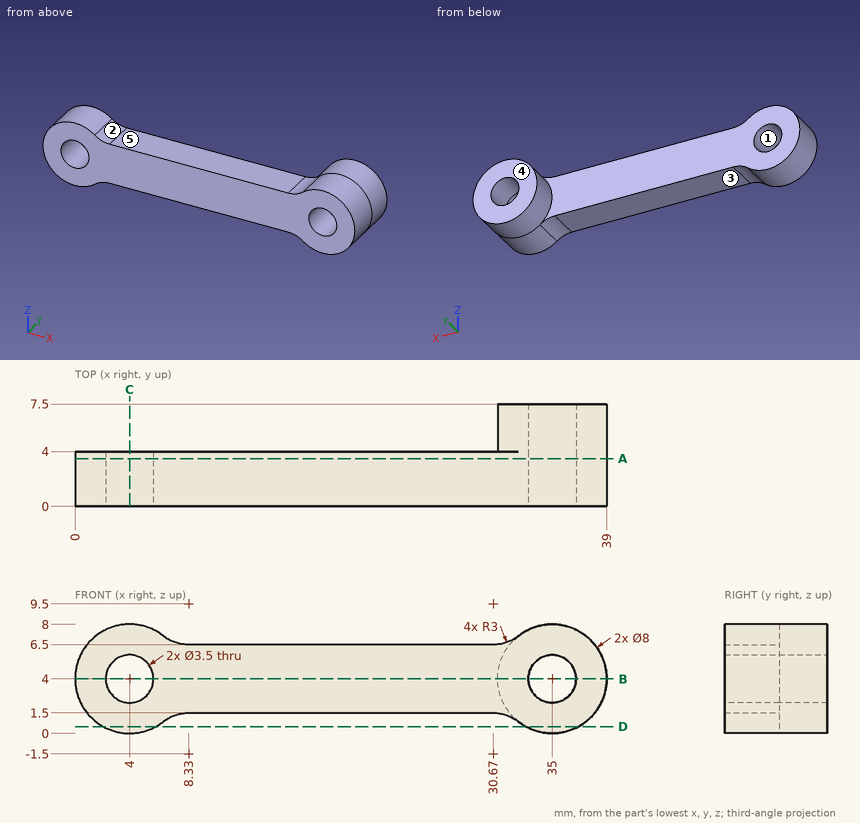
The figure shows three views and two pictorial views of one solid part (mm, origin at its lowest corner). Answer the questions. A direction names the side the tool comes from. Round coordinates to 2 decimals unless told otherwise and drop trailing zeros. Write each loop counter-clockwise with the first axis right and the second up, starting at its lowest first coordinate (ties: lowest second). Pieces come first, ordered by that corner, then holes. Notation, with made-up numbers: (15.5, 59.5) - (71.5, 59.5) arc R23 cw to (71.5, 72.5) - close; hole circle Ø7 at (1.25, 26.25). An arc over 180 degrees is marked (long way). One line per question, with ' | ' between items. Start each with the question number.
1. Section D-D (z = 0.5) is taken. Determine the outline of the cut face in (x, y), and give its area (3 significant figures).
2. Section A-A (y = 3.5) is taken. Determine the outline of the cut face in (x, z).
3. For a pull along X with two mould halves and no side action, classify the marked faces 4 and 5 as +X half, -X half, draft (parallel to the pull), parting line (faces both ways), or undercut.
4. Each of these flat-tipped pins is pushed along its axis until it touches: pin 1 (4.5 mm diameter, centred on x = 17, y = 1.5, fed in from -Z); pin 2 (4.5 mm diameter, centred on x = 17.5, y = 1, fed in from +Z). Where does it stop, or does it pass through?
5. Section B-B (z = 4) is taken. Determine the outline of the cut face in (x, y), and give its area (3 significant figures).
6. For the marked faces 1, 2 and 3, determine the directions among +Z, -Z, +X, -X, +Y, -Y from which every point of the face is accessible in a straight line to the end or side of a thin tool.
7. Find the intervals of material crossed by probe 1 along Z at (x, y) = (35, 4); probe 2 along X at (y, z) = (3.25, 3); probe 3 along Y at (x, z) = (25.5, 2), in increasing order. Write a range as [from, to].
8. Section C-C (x = 4) is taken. Determine the outline of the cut face in (y, z), and give its area (3 significant figures).
Filled in:
1) outline: (2.06, 0) - (5.94, 0) - (5.94, 4) - (2.06, 4) - close; (33.06, 0) - (36.94, 0) - (36.94, 7.5) - (33.06, 7.5) - close | area: 44.5 mm²
2) outline: (6.47, 0.86) arc R3 cw to (8.33, 1.5) - (30.67, 1.5) arc R3 cw to (32.53, 0.86) arc R4 ccw (long way) to (32.53, 7.14) arc R3 cw to (30.67, 6.5) - (8.33, 6.5) arc R3 cw to (6.47, 7.14) arc R4 ccw (long way) to start; hole circle Ø3.5 at (4, 4); hole circle Ø3.5 at (35, 4)
3) face 4: draft | face 5: undercut
4) pin 1: z = 1.5 | pin 2: z = 6.5
5) outline: (0, 0) - (2.25, 0) - (2.25, 4) - (0, 4) - close; (5.75, 0) - (33.25, 0) - (33.25, 7.5) - (31, 7.5) - (31, 4) - (5.75, 4) - close; (36.75, 0) - (39, 0) - (39, 7.5) - (36.75, 7.5) - close | area: 144 mm²
6) face 1: +Y, -Y | face 2: +Z, +Y, -Y | face 3: -Z, +Y, -Y
7) probe 1: [0, 2.25], [5.75, 8] | probe 2: [0.13, 2.56], [5.44, 33.56], [36.44, 38.87] | probe 3: [0, 4]
8) outline: (0, 0) - (4, 0) - (4, 2.25) - (0, 2.25) - close; (0, 5.75) - (4, 5.75) - (4, 8) - (0, 8) - close | area: 18.0 mm²
